from build123d import *

# Parameters (mm, degrees)
SKETCH1_R           = 5
BOSS_EXTRUDE1_DEPTH = 2.5
SKETCH6_W           = 0.25
SKETCH6_H           = 1
BOSS_EXTRUDE4_DEPTH = 2.5
CIRPATTERN1_COUNT   = 4
SKETCH8_R           = 2.5
CUT_EXTRUDE3_DEPTH  = 1.25
SKETCH9_W           = 1
SKETCH9_H           = 1.35
BOSS_EXTRUDE5_DEPTH = 9.5
SKETCH11_R          = 3.85
CUT_EXTRUDE4_DEPTH  = 14
SKETCH12_R          = 0.48
BOSS_EXTRUDE6_DEPTH = 7
SKETCH13_R          = 3.75
CUT_EXTRUDE5_DEPTH  = 7
CUT_EXTRUDE6_START  = 17
SKETCH14_R          = 6.794989929
SKETCH14_R_2        = 5
CUT_EXTRUDE6_DEPTH  = 17


with BuildPart() as part:
    # Sketch1 → Boss-Extrude1 (new body)
    with BuildSketch(Plane.XY):
        Circle(SKETCH1_R)
    extrude(amount=BOSS_EXTRUDE1_DEPTH)

    # Sketch6 → Boss-Extrude4 (add)
    with BuildSketch(Plane.XY.offset(2.5)):
        with Locations((-5.025, 0)):
            Rectangle(SKETCH6_W, SKETCH6_H)
    boss_extrude4 = extrude(amount=-BOSS_EXTRUDE4_DEPTH)

    # CirPattern1: Boss-Extrude4 ×4 about axis
    cirpattern1_axis = Axis((0, 0, 0), (0, 0, 1))
    for i in range(1, CIRPATTERN1_COUNT):
        add(boss_extrude4.rotate(cirpattern1_axis, i * 360 / CIRPATTERN1_COUNT))

    # Sketch8 → Cut-Extrude3 (cut)
    with BuildSketch(Plane.XY.offset(2.5)):
        Circle(SKETCH8_R)
    extrude(amount=-CUT_EXTRUDE3_DEPTH, mode=Mode.SUBTRACT)

    # Sketch9 → Boss-Extrude5 (add)
    with BuildSketch(Plane(origin=(0, 0, 0), x_dir=(-1, 0, 0), z_dir=(0, 0, -1))):
        with Locations((0, 4.475)):
            Rectangle(SKETCH9_W, SKETCH9_H)
    extrude(amount=BOSS_EXTRUDE5_DEPTH)

    # Sketch11 → Cut-Extrude4 (cut)
    with BuildSketch(Plane(origin=(0, 0, 0), x_dir=(-1, 0, 0), z_dir=(0, 0, -1))):
        Circle(SKETCH11_R)
    extrude(amount=CUT_EXTRUDE4_DEPTH, mode=Mode.SUBTRACT)

    # Sketch12 → Boss-Extrude6 (add)
    with BuildSketch(Plane(origin=(0, 5.15, 0), x_dir=(1, 0, 0), z_dir=(0, 1, 0))):
        with Locations(Location((0, 8.9, 0), (0, 0, 180))):
            Circle(SKETCH12_R)
    extrude(amount=-BOSS_EXTRUDE6_DEPTH)

    # Sketch13 → Cut-Extrude5 (cut)
    with BuildSketch(Plane(origin=(0, 0, -9.5), x_dir=(-1, 0, 0), z_dir=(0, 0, -1))):
        Circle(SKETCH13_R)
    extrude(amount=-CUT_EXTRUDE5_DEPTH, mode=Mode.SUBTRACT)

    # Sketch14 → Cut-Extrude6 (cut)
    with BuildSketch(Plane(origin=(0, 0, 0), x_dir=(-1, 0, 0), z_dir=(0, 0, -1)).offset(CUT_EXTRUDE6_START)):
        Circle(SKETCH14_R)
        Circle(SKETCH14_R_2, mode=Mode.SUBTRACT)
    extrude(amount=-CUT_EXTRUDE6_DEPTH, mode=Mode.SUBTRACT)


solid = part.part
Geometry: final body of the model. Coordinates: model frame, mm. A direction names the side the tool comes from. Round coordinates to 2 decimals unless told otherwise and drop trailing zeros. Write each loop counter-clockwise with the first axis right and the second up, starting at its lowest first coordinate (ties: lowest second). Pieces come first, ordered by that corner, then holes. Notation, with made-up numbers: M 70,19.25 L 110,19.25 A16 cw 110,50.25 Z; hole C -15.75,36 d5. An arc over 180 degrees is marked long. Write item = value, one per line.
Item 1: Section query A-A on z = 1. Return loops of the section in (x, y), then the cut area to 3 significant figures.
Findings:
outline = M -5.15,-0.5 L -4.97,-0.5 A5 ccw -0.5,-4.97 L -0.5,-5.15 L 0.5,-5.15 L 0.5,-4.97 A5 ccw 4.97,-0.5 L 5.15,-0.5 L 5.15,0.5 L 4.97,0.5 A5 ccw 0.5,4.97 L 0.5,5.15 L -0.5,5.15 L -0.5,4.97 A5 ccw -4.97,0.5 L -5.15,0.5 Z
area = 79.2 mm^2
Item 2: Section query B-B on x = 0. Return loops of the section in (y, z), then the cut area to 3 significant figures.
Findings:
outline = M -5.15,0 L 3.85,0 L 3.85,-8.42 L 3.75,-8.42 L 3.75,-9.38 L 3.85,-9.38 L 3.85,-9.5 L 5,-9.5 L 5,0 L 5.15,0 L 5.15,2.5 L 2.5,2.5 L 2.5,1.25 L -2.5,1.25 L -2.5,2.5 L -5.15,2.5 Z
area = 30.5 mm^2
Item 3: Section query C-C on y = 0. Return loops of the section in (x, z).
Findings:
outline = M -5.15,0 L 5.15,0 L 5.15,2.5 L 2.5,2.5 L 2.5,1.25 L -2.5,1.25 L -2.5,2.5 L -5.15,2.5 Z
Item 4: Material intervals for line 1 along Y through (x, z) = (0, 1.75); line 2 along Z through (x, y) = (-3, -1.5); line 3 along Z through (x, y) = (-1, 1), sorted ascending. Write a range as [from, to].
Findings:
line_1 = [-5.15, -2.5], [2.5, 5.15]
line_2 = [0, 2.5]
line_3 = [0, 1.25]
Item 5: Pull-direction query (Y, two-part tool) for faces 5 (the face through (-3.57, -3.5, 1.23)), 6 (the face through (0, 0, 1.25)), 7 (the face through (0, 0, 0)); classes: pulls with the +Y half, pulls with the -Y half, needs draft (parallel to the pull), parting line crosses it, or undercut.
Findings:
face_5 = pulls with the -Y half
face_6 = undercut
face_7 = needs draft
Item 6: Access query for faces 1 (the face through (-0.01, 3.85, -4.68)), 2 (the face through (0.5, 4, -5)), 3 (the face through (-0.5, 4, -5)), 4 (the face through (-0.54, -2.44, 1.88)). Directions: +Z, -Z, +X, -X, +Y, -Y. A direction counts if a zero-diameter tool reaches every point of the face in a straight line with its end or side. Return the directions, or none.
Findings:
face_1 = -Y
face_2 = -Z, +X, +Y, -Y
face_3 = -Z, -X, +Y, -Y
face_4 = +Z
Item 7: Pin query (flat end, axial travel): P1, Ø3, axis at x = 0, y = 0, coming from the +Z side; P2, Ø1.3, axis at y = 4.5, z = -7, coming from the -X side; P3, Ø3, axis at y = 2.5, z = -3, coming from the +X side. Return the tip coordinate at first contact, or that it passes through.
Findings:
P1 = 1.25
P2 = -0.5
P3 = 0.5
